from build123d import *

# Parameters (mm, degrees)
BOSS_EXTRUDE1_DEPTH = 45.72
SKETCH5_R           = 6.0198
BOSS_EXTRUDE3_DEPTH = 14.732
BOSS_EXTRUDE4_DEPTH = 6.4516


with BuildPart() as part:
    # Sketch2 → Boss-Extrude1 (new body)
    with BuildSketch(Plane.XY):
        Polygon((0, 8.62284174), (-7.4676, 4.31142087), (-7.4676, -4.31142087), (0, -8.62284174), (7.4676, -4.31142087), (7.4676, 4.31142087), align=None)
    extrude(amount=BOSS_EXTRUDE1_DEPTH)

    # Sketch1 → Cut-Revolve1 (revolve, cut)
    with BuildSketch(Plane(origin=(0, 0, 0), x_dir=(0, 0, -1), z_dir=(1, 0, 0)), mode=Mode.PRIVATE) as cut_revolve1_sk:
        Polygon((8.722264365, 0), (8.722264365, 28.967330829), (-61.313897387, 28.967330829), (-61.313897387, 0), (-28.3972, 0), (-28.3972, 4.523893796), (-37.4396, 5.1562), (-37.4396, 6.1468), (-35.9156, 6.1468), (-35.9156, 6.7564), (-25.4, 6.7564), (-25.4, 17.888200709), (-12.872167857, 17.888200709), (-9.0424, 7.366), (-9.0424, 5.1562), (0, 4.523893796), (0, 2.5781), (-2.5781, 2.5781), (-2.5781, 0), align=None)
    revolve(cut_revolve1_sk.sketch.rotate(Axis((0, 0, -8.722264365), (0, 0, -1)), 90), axis=Axis((0, 0, -8.722264365), (0, 0, -1)), mode=Mode.SUBTRACT)

    # Sketch4 → Revolve1 (revolve)
    with BuildSketch(Plane(origin=(0, 0, 0), x_dir=(0, 0, -1), z_dir=(1, 0, 0)), mode=Mode.PRIVATE) as revolve1_sk:
        Polygon((-25.4, 8.82604174), (-24.384, 8.82604174), (-19.479330617, 3.921372357), (-25.4, 3.921372357), align=None)
    revolve(revolve1_sk.sketch.rotate(Axis((0, 0, 13.232415159), (0, 0, -1)), 90), axis=Axis((0, 0, 13.232415159), (0, 0, -1)))

    # Sketch5 → Boss-Extrude3 (add)
    with BuildSketch(Plane(origin=(0, 0, 0), x_dir=(1, 0, 0), z_dir=(0, 1, 0))):
        with Locations(Location((0, -15.748, 0), (0, 0, 270))):
            Circle(SKETCH5_R)
    extrude(amount=BOSS_EXTRUDE3_DEPTH)

    # Sketch6 → Boss-Extrude4 (add)
    with BuildSketch(Plane(origin=(0, 14.732, 0), x_dir=(1, 0, 0), z_dir=(0, 1, 0))):
        with BuildLine():
            Line((-2.796240531, -21.7932), (16.8402, -21.7932))
            ThreePointArc((16.8402, -21.7932), (18.277040979, -21.198040979), (18.8722, -19.7612))
            Line((18.8722, -19.7612), (18.8722, -11.7348))
            ThreePointArc((18.8722, -11.7348), (18.277040979, -10.297959021), (16.8402, -9.7028))
            Line((16.8402, -9.7028), (-2.796240531, -9.7028))
            ThreePointArc((-2.796240531, -9.7028), (-3.559009839, -9.851396968), (-4.210218905, -10.275454545))
            ThreePointArc((-4.210218905, -10.275454545), (-6.5278, -15.748), (-4.210218905, -21.220545455))
            ThreePointArc((-4.210218905, -21.220545455), (-3.559009839, -21.644603032), (-2.796240531, -21.7932))
        make_face()
    extrude(amount=BOSS_EXTRUDE4_DEPTH)


solid = part.part
Input: part model. Units: mm. Frame: model coordinates. A direction names the side the tool comes from. Give positions to 0.01 mm unless a question says otherwise; leave off trailing zeros. Order: outer loops, then holes, each group sorted by start corner. A loop starts at its lowest first (then second) coordinate and runs counter-clockwise, first axis right, second up. Notation, with made-up numbers: (56, 14.5) - (72, 14.5) arc R20 ccw to (72, 22.5) - close; hole circle Ø3 at (-40, 79). An arc over 180 degrees is marked (long way). Write each question's results on one line, items separated by ' | '.
Item 1: Section D-D (x = 9.5). Return loops of the section in (y, z).
A:
outline: (14.73, 9.7) - (21.18, 9.7) - (21.18, 21.79) - (14.73, 21.79) - close
Item 2: Material intervals for line 1 along Y through (x, z) = (0, 1.6); line 2 along Z through (x, y) = (6, 3); line 3 along Z through (x, y) = (-1, -1), sorted ascending.
A:
line 1: y = -4.64 to -2.58, 2.58 to 4.64 | line 2: z = 9.04 to 35.92 | line 3: z = 2.58 to 28.4
Item 3: Section A-A (y = 17). Return loops of the section in (x, z), and give its area (3 significant figures).
A:
outline: (-4.21, 10.28) arc R2.03 ccw to (-2.8, 9.7) - (16.84, 9.7) arc R2.03 ccw to (18.87, 11.73) - (18.87, 19.76) arc R2.03 ccw to (16.84, 21.79) - (-2.8, 21.79) arc R2.03 ccw to (-4.21, 21.22) arc R7.62 ccw to start | area: 294 mm^2
Item 4: Section B-B (z = 22.5). Return loops of the section in (x, y).
A:
outline: (-7.47, -4.31) - (0, -8.62) - (7.47, -4.31) - (7.47, 4.31) - (0, 8.62) - (-7.47, 4.31) - close
Item 5: Contact query for flat-ended pins moving along their axis: pin 1 Ø1.9 at (x, y) = (9, 18.5) entering from +Z; pin 2 Ø7 at (y, z) = (0, 16.5) entering from +X; pin 3 Ø8 at (y, z) = (16, 21) entering from -X; pin 4 Ø5.5 at (x, y) = (-3, -2) entering from +Z. Output: stop coordinate, or through.
A:
pin 1: stops at z = 21.79 | pin 2: stops at x = 7.47 | pin 3: stops at x = -6.42 | pin 4: stops at z = 37.44
Item 6: Access query for faces 1 (the flat face through (-5, 5, 25.4)), 2 (the cylindrical face through (-6.527, 17.913, 15.663)), 3 (the flat face through (7, 18, 21.793)), 4 (the cylindrical face through (-0.336, -2.556, 1.307)). Directions: +Z, -Z, +X, -X, +Y, -Y. A direction counts if a zero-diameter tool reaches every point of the face in a straight line with its end or side. Return the directions, or none.
A:
face 1: +Z | face 2: -X, +Y | face 3: +Z, +X, -X, +Y | face 4: -Z
Item 7: Draft query along Z for faces 5 (the flat face through (2, 6, 35.916)), 6 (the conical face through (4.13, -6.48, 23.24)), 7 (the flat face through (2, 2, 0)), 8 (the flat face through (-3.786, -6.437, 16.524)). Return one class per face: released by +Z, released by -Z, zero draft, split by the parting line, or undercut.
A:
face 5: released by +Z | face 6: undercut | face 7: released by -Z | face 8: zero draft
